Geometry check sheet. Reference: the model listing, model coordinates, mm. Face numbers are marked on the shaded views. A direction names the side the tool comes from. Give positions to 0.01 mm unless a question says otherwise; leave off trailing zeros. Order: outer loops, then holes, each group sorted by start corner. A loop starts at its lowest first (then second) coordinate and runs counter-clockwise, first axis right, second up. Notation, with made-up numbers: M 38,71.5 L 79,71.5 A26 cw 79,86.5 Z; hole C 59,-28 d10. An arc over 180 degrees is marked long. Answer as CSV lines item,"result". Start each with the question number.
Q1. Go/stop test with flat-tipped pins: pin 1 (12 mm diameter, centred on x = 5.5, y = 15.5, fed in from +Z); pin 2 (8.5 mm diameter, centred on y = 0, z = 0, fed in from +X); pin 3 (8 mm diameter, centred on x = 2.5, z = 7, fed in from +Y); pin 4 (1 mm diameter, centred on x = 17, z = -10, fed in from +Y). Record where each tip stops, or that it passes through.
Q2. Section check A-A, the plane y = 0. Record the boundary of the cut face in (x, z), then the cut area to 3 significant figures.
Q3. Section check C-C, the plane x = 1. Record the boundary of the cut face in (y, z).
Q4. Thickness scan on line 1 (X direction, y = 11, z = -13); line 2 (X direction, y = -9, z = -20.5); line 3 (Z direction, x = 9, y = -5). Record the ranges inside material, lowest first.
Q5. Set-up check for the marked faces 1 and 2: record each of +Z, -Z, +X, -X, +Y, -Y from which the full face is reachable in a straight line by a thin tool's end or side.
Q6. Mould release check, pull along Y, two halves, no side actions. Record for the marked faces 3, 4 and 5: +Y half, -Y half, draft (parallel to the pull), parting line (faces both ways), or undercut.
Autodesk Inventor part; units mm, degrees
ref_plane "YZ Plane" through (0, 0, 0) normal (1, 0, 0) x (0, 1, 0)
ref_plane "XZ Plane" through (0, 0, 0) normal (0, 1, 0) x (-1, 0, 0)
ref_plane "XY Plane" through (0, 0, 0) normal (0, 0, 1) x (1, 0, 0)
sketch "Sketch1" plane through (0, 0, 0) normal (1, 0, 0) x (0, 1, 0)
  circle A0 centre (0, 0) radius 28
  dimension "d0" = 56
extrude "Extrusion1" add sketch "Sketch1" along normal blind 24
sketch "Sketch2" plane through (24, 0, 0) normal (1, 0, 0) x (0, 0, -1)
  circle A0 centre (0, 0) radius 13
  dimension "d3" = 26
extrude "Extrusion2" add sketch "Sketch2" along normal blind 2
sketch "Sketch3" plane through (0, 0, 0) normal (-1, 0, 0) x (0, 0, 1)
  circle A0 centre (0, 0) radius 13
  dimension "d6" = 26
extrude "Extrusion3" add sketch "Sketch3" along normal blind 2
sketch "Sketch8" plane through (0, 0, 0) normal (0, 0, 1) x (1, 0, 0)
  line L0 (0, 28) -> (24, 28)
  circle A0 centre (12, 28) radius 7
  line L1 (-19.1925, 0) -> (68.2113, 0)
  point P0 (0, 0)
  dimension "d14" = 14
revolve "Revolution1" cut sketch "Sketch8" angle 360 about axis through (-19.1925, 0, 0) along (1, 0, 0)
sketch "Sketch9" plane through (26, 0, 0) normal (1, 0, 0) x (0, 0, -1)
  circle A0 centre (0, 0) radius 7
  dimension "d16" = 14
extrude "Extrusion4" cut sketch "Sketch9" against normal blind 30
properties part number "Roue" material "Aluminum 6061-AHC"
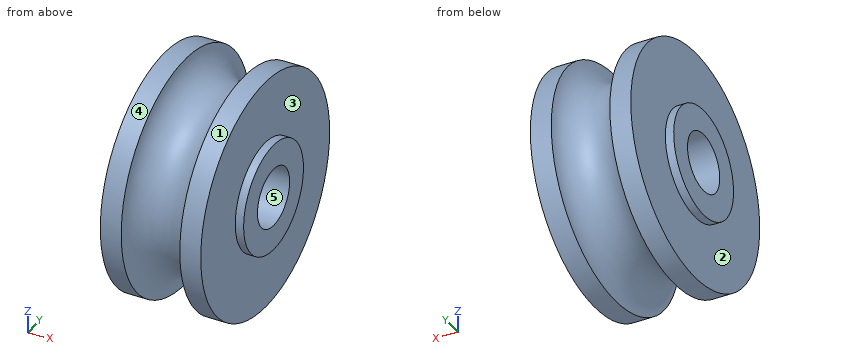
Answer block:
1,pin 1,"stops at z = 26.33"
1,pin 2,"passes through"
1,pin 3,"stops at y = 27.84"
1,pin 4,"stops at y = 21.49"
2,outline,"M -2,-13 L 0,-13 L 0,-28 L 5,-28 A7 cw 19,-28 L 24,-28 L 24,-13 L 26,-13 L 26,-7 L -2,-7 Z; M -2,7 L 26,7 L 26,13 L 24,13 L 24,28 L 19,28 A7 cw 5,28 L 0,28 L 0,13 L -2,13 Z"
2,area,"902 mm2"
3,outline,"C 0,0 d56; hole C 0,0 d14"
4,line 1,"x = 0 to 24"
4,line 2,"x = 0 to 7.82, 16.18 to 24"
4,line 3,"z = -21.09 to -4.9, 4.9 to 21.09"
5,face 1,"+X, -X"
5,face 2,"-X"
6,face 3,"draft"
6,face 4,"parting line"
6,face 5,"undercut"
